```python
from build123d import *

# Parameters (mm, degrees)
F1_DEPTH = 110.000034
F2_W     = 110
F2_H     = 379.99924
F3_DEPTH = 270
F5_DEPTH = 110
F6_W     = 380
F6_H     = 80
F7_DEPTH = 380
F9_DEPTH = 80


with BuildPart() as f1:
    # F0 (on Top) → F1 (new body)
    with BuildSketch(Plane.XY):
        with BuildLine():
            ThreePointArc((189.99962, -189.99962), (0, 0), (189.99962, 189.99962))
            Line((189.99962, 189.99962), (-189.99962, 189.99962))
            Line((-189.99962, 189.99962), (-189.99962, -189.99962))
            Line((-189.99962, -189.99962), (189.99962, -189.99962))
        make_face()
        with BuildLine():
            ThreePointArc((379.99924, 0), (324.34964, 134.35002), (189.99962, 189.99962))
            Line((189.99962, 189.99962), (189.99962, -189.99962))
            ThreePointArc((189.99962, -189.99962), (324.34964, -134.35002), (379.99924, 0))
        make_face()
        with BuildLine():
            Line((189.99962, -189.99962), (189.99962, 189.99962))
            ThreePointArc((189.99962, 189.99962), (0, 0), (189.99962, -189.99962))
        make_face()
    extrude(amount=F1_DEPTH)

    # F2 (on face) → F3 (join)
    with BuildSketch(Plane.XY.offset(110.000034)):
        with Locations((-134.99962, 0)):
            Rectangle(F2_W, F2_H)
    extrude(amount=F3_DEPTH)

    # F4 (on face) → F5 (join)
    with BuildSketch(Plane(origin=(-189.99962, 0, 0), x_dir=(0, -1, 0), z_dir=(-1, 0, 0))):
        with BuildLine():
            Line((-189.99962, 380.000034), (189.99962, 380.000034))
            ThreePointArc((189.99962, 380.000034), (0, 569.99924), (-189.99962, 380.000034))
        make_face()
    extrude(amount=-F5_DEPTH)

    # F6 (on face) → F7 (join)
    with BuildSketch(Plane.XY.offset(110.000034)):
        with Locations((110.00038, -0.00038)):
            Rectangle(F6_W, F6_H)
    extrude(amount=F7_DEPTH)

    # F8 (on face) → F9 (cut, through all)
    with BuildSketch(Plane.XZ.offset(40.00038)):
        Polygon((300.00038, 490.000034), (-79.99962, 490.000034), (300.00038, 110.000034), align=None)
    extrude(amount=-F9_DEPTH, mode=Mode.SUBTRACT)


solid = f1.part
```
Source: CAD feature listing. Evaluate the final solid. Frame: model axes, mm. A direction names the side the tool comes from. Round coordinates to 2 decimals unless told otherwise and drop trailing zeros. Write each loop counter-clockwise with the first axis right and the second up, starting at its lowest first coordinate (ties: lowest second). Pieces come first, ordered by that corner, then holes. Notation, with made-up numbers: M -18.75,-7.75 L -9.75,-7.75 A38 cw -9.75,31.25 Z; hole C 69.5,41.25 d11. An arc over 180 degrees is marked long. Use CSV: the item, a comma, the result in double quotes. Start each with the question number.
Q1. Line query: line 1 (Z direction, x = 31, y = 103); line 2 (X direction, y = 151.5, z = 485); line 3 (Y direction, x = 126, z = 130). Output: solid intervals per line, ascending. Write a range as from..to.
Q2. First-contact query: P1, Ø4, axis at x = -87.5, y = -38.5, coming from the +Z side; P2, Ø10, axis at x = 31, z = 324, coming from the +Y side; P3, Ø6, axis at x = 117.5, z = 217.5, coming from the -Y side. Flat tips, straight axial feed; report the tip coordinate or a pass-through.
Q3. Cut plane A-A on x = 214.5. Output: boundary loops of the cut face in (y, z).
Q4. Cut plane D-D on x = -128. Output: boundary loops of the cut face in (y, z), plus the area to 3 significant figures.
Q5. Cut plane C-C on z = 237.5. Output: boundary loops of the cut face in (x, y), plus the area to 3 significant figures.
Q6. Cut plane B-B on y = 63.5. Output: boundary loops of the cut face in (x, z), plus the area to 3 significant figures.
Q7. Access query for faces 1 (the face through (-80, 45, 343)), 2 (the face through (65, -40, 255)), 3 (the face through (107, -1, 303)), 4 (the face through (65, 40, 255)), 5 (the face through (-87, -190, 145)). Directions: +Z, -Z, +X, -X, +Y, -Y. A direction counts if a zero-diameter tool reaches every point of the face in a straight line with its end or side. Return the directions, or none.
Results found:
1,line 1,"0..110"
1,line 2,"-190..-80"
1,line 3,"-40..40"
2,P1,"z = 566.46"
2,P2,"y = 40"
2,P3,"y = -40"
3,outline,"M -188.41,0 L 188.41,0 L 188.41,110 L 40,110 L 40,195.5 L -40,195.5 L -40,110 L -188.41,110 Z"
4,outline,"M -190,0 L 190,0 L 190,380 A190 ccw -190,380 Z"
4,area,"201,000 mm^2"
5,outline,"M -190,-190 L -80,-190 L -80,-40 L 172.5,-40 L 172.5,40 L -80,40 L -80,190 L -190,190 Z"
5,area,"62,000 mm^2"
6,outline,"M -190,0 L 369.07,0 L 369.07,110 L -80,110 L -80,559.07 L -190,559.07 Z"
6,area,"111,000 mm^2"
7,face 1,"+Z, +X"
7,face 2,"+Z, +X, -Y"
7,face 3,"+Z, +X, +Y, -Y"
7,face 4,"+Z, +X, +Y"
7,face 5,"+Z, -Z, +X, -X, -Y"
